Source: CAD feature listing. Evaluate the final solid. Frame: model axes, mm. A direction names the side the tool comes from. Round coordinates to 2 decimals unless told otherwise and drop trailing zeros. Loops run counter-clockwise (first coordinate to the right, second up) from the corner with the lowest first, then second, coordinate; pieces in that order, holes last. Notation, with made-up numbers: M 51.25,42.25 L 90.25,42.25 A20 cw 90.25,73.25 Z; hole C 72.5,83 d7. An arc over 180 degrees is marked long. Answer as CSV lines item,"result". Start each with the question number.
```python
from build123d import *

# Parameters (mm, degrees)
F0_R     = 10.9
F1_DEPTH = 70
F5_R     = 4.85
F6_DEPTH = 6.5


with BuildPart() as f1:
    # F0 (on Top) → F1 (new body)
    with BuildSketch(Plane.XY):
        Circle(F0_R)
    extrude(amount=F1_DEPTH)

    # F2 (on Front) → F3 (revolve, cut)
    with BuildSketch(Plane.XZ):
        with BuildLine():
            Line((0, 41.7), (0, 0))
            Line((0, 0), (10.5, 0))
            ThreePointArc((10.5, 0), (7.947904, 4.964478), (3.8, 8.7))
            Line((3.8, 8.7), (3.8, 41.7))
            Line((3.8, 41.7), (0, 41.7))
        make_face()
    revolve(axis=Axis((0, 0, 20.85), (0, 0, -1)), mode=Mode.SUBTRACT)

    # F5 (on offset) → F6 (join)
    with BuildSketch(Plane.XY.offset(70)):
        Circle(F5_R)
    extrude(amount=F6_DEPTH)


solid = f1.part
```
1) Contact query for flat-ended pins moving along their axis: pin 1 Ø2 at (y, z) = (1, 15.5) entering from -X; pin 2 Ø1 at (x, z) = (7, 53.5) entering from -Y; pin 3 Ø2.5 at (x, y) = (0, 1.5) entering from -Z; pin 4 Ø5 at (x, y) = (3.5, -5) entering from -Z. Output: stop coordinate, or through.
2) Ray query, line 1 along Y through (x, z) = (0, 28.5); line 2 along X through (y, z) = (1.5, 4.5); line 3 along Y through (x, z) = (-1.25, 9). Return the intervals inside material, ascending.
3) Mould query, pull axis Y, two halves, no side actions, for faces 4 (the cylindrical face through (-3.796, -0.167, 25.431)), 5 (the flat face through (0, 0, 76.5)), 6 (the cylindrical face through (4.626, 1.457, 73.204)). Classes: pulls with the +Y half, pulls with the -Y half, needs draft (parallel to the pull), parting line crosses it, or undercut.
4) Section A-A, the plane z = 19. Return loops of the section in (x, y).
5) Access query for faces 1 (the cylindrical face through (10.4, 3.27, 34.51)), 2 (the flat face through (0, 0, 41.7)), 3 (the flat face through (2, -5, 70)). Directions: +Z, -Z, +X, -X, +Y, -Y. A direction counts if a zero-diameter tool reaches every point of the face in a straight line with its end or side. Return the directions, or none.
Findings below:
1,pin 1,"x = -10.9"
1,pin 2,"y = -8.75"
1,pin 3,"z = 41.7"
1,pin 4,"z = 4.05"
2,line 1,"-10.9 to -3.8, 3.8 to 10.9"
2,line 2,"-10.8 to -8.16, 8.16 to 10.8"
2,line 3,"-10.83 to -3.59, 3.59 to 10.83"
3,face 4,"undercut"
3,face 5,"needs draft"
3,face 6,"parting line crosses it"
4,outline,"C 0,0 d21.8; hole C 0,0 d7.6"
5,face 1,"+Z, -Z"
5,face 2,"-Z"
5,face 3,"+Z"
